Design review of the part built by this model. Coordinates are the model's own, in mm. A direction names the side the tool comes from. Give positions to 0.01 mm unless a question says otherwise; leave off trailing zeros. Order: outer loops, then holes, each group sorted by start corner. A loop starts at its lowest first (then second) coordinate and runs counter-clockwise, first axis right, second up. Notation, with made-up numbers: (73.5, 49) -> (127.5, 49) arc R28 cw to (127.5, 76) -> close; hole circle Ø10 at (-23, -29.5). An arc over 180 degrees is marked (long way). One line per item, written item: value. Start each with the question number.
1) Consider section A-A (z = 13). State the section outline as (x, y) points.
2) Wall thickness on line 1 along Y through (x, z) = (6.5, 45); line 2 along X through (y, z) = (-27, 34); line 3 along Z through (x, y) = (-24, 22.5): over which ranges is each line inside the solid? List them lowest first. Write a range as from..to.
3) Tool access review of faces 1 (the face through (1, 47.5, 26)), 2 (the face through (-1, 1, 0)): name each direction out of +Z, -Z, +X, -X, +Y, -Y from which nothing blocks a thin tool from reaching the whole face with its end or side.
4) Consider section C-C (y = 7). State the section outline as (x, z) points, plus the area to 4 significant figures.
5) For pin 1 (3 mm diameter, centred on x = 17, y = -28, fed in from +Z), flat-tipped, find the tip position at first contact; note if it passes through.
6) The part is to be moulded in two halves that separate along X. For faces 3 (the face through (-1, -47.5, 26)), 4 (the face through (1, 50, 25)), 5 (the face through (72.15, 46.99, 24.65)), say which applies: released by +X, released by -X, zero draft, split by the parting line, or undercut.
7) Consider section B-B (x = -34). State the section outline as (y, z) points.
from build123d import *

# Parameters (mm, degrees)
F1_DEPTH = 50
F2_T     = -2.5


with BuildPart() as f1:
    # F0 (on Top) → F1 (new body)
    with BuildSketch(Plane.XY):
        with BuildLine():
            Line((-65, -50), (65, -50))
            ThreePointArc((65, -50), (72.071068, -47.071068), (75, -40))
            Line((75, -40), (75, 40))
            ThreePointArc((75, 40), (72.071068, 47.071068), (65, 50))
            Line((65, 50), (-65, 50))
            ThreePointArc((-65, 50), (-72.071068, 47.071068), (-75, 40))
            Line((-75, 40), (-75, -40))
            ThreePointArc((-75, -40), (-72.071068, -47.071068), (-65, -50))
        make_face()
    extrude(amount=F1_DEPTH)

    # F2
    f2_openings = [f1.faces().sort_by_distance(p)[0] for p in [
        (0, 0, 50),
    ]]
    offset(amount=F2_T, openings=f2_openings)


solid = f1.part
Checked values:
1. outline: (-75, -40) arc R10 ccw to (-65, -50) -> (65, -50) arc R10 ccw to (75, -40) -> (75, 40) arc R10 ccw to (65, 50) -> (-65, 50) arc R10 ccw to (-75, 40) -> close; hole (-72.5, -40) arc R7.5 ccw to (-65, -47.5) -> (65, -47.5) arc R7.5 ccw to (72.5, -40) -> (72.5, 40) arc R7.5 ccw to (65, 47.5) -> (-65, 47.5) arc R7.5 ccw to (-72.5, 40) -> close
2. line 1: y = -50..-47.5, 47.5..50
2. line 2: x = -75..-72.5, 72.5..75
2. line 3: z = 0..2.5
3. face 1: +Z
3. face 2: -Z, +X, -X, +Y, -Y
4. outline: (-75, 0) -> (75, 0) -> (75, 50) -> (72.5, 50) -> (72.5, 2.5) -> (-72.5, 2.5) -> (-72.5, 50) -> (-75, 50) -> close
4. area: 612.5 mm^2
5. pin 1: stops at z = 2.5
6. face 3: undercut
6. face 4: zero draft
6. face 5: released by +X
7. outline: (-50, 0) -> (50, 0) -> (50, 50) -> (47.5, 50) -> (47.5, 2.5) -> (-47.5, 2.5) -> (-47.5, 50) -> (-50, 50) -> close
